Geometry check sheet. Reference: the model listing, model coordinates, mm. Round coordinates to 2 decimals unless told otherwise and drop trailing zeros. Loops run counter-clockwise (first coordinate to the right, second up) from the corner with the lowest first, then second, coordinate; pieces in that order, holes last. Notation, with made-up numbers: (-21.75, -12) - (-8.75, -12) arc R27 ccw to (-8.75, 13) - close; hole circle Ø3 at (42, -28). An arc over 180 degrees is marked (long way). Write item = value, one per line.
```python
from build123d import *

# Parameters (mm, degrees)
SKETCH1_R           = 2.75
BOSS_EXTRUDE1_DEPTH = 5.5


with BuildPart() as part:
    # Sketch1 → Boss-Extrude1 (new body)
    # profile 1 of 3: a face of its own
    with BuildSketch(Plane.XY):
        with BuildLine():
            ThreePointArc((-12.496095275, 0.312414586), (0, 12.5), (12.496095275, 0.312414586))
            Line((12.496095275, 0.312414586), (7.499414268, 400.093731696))
            ThreePointArc((7.499414268, 400.093731696), (0, 407.5), (-7.499414268, 400.093731696))
            Line((-7.499414268, 400.093731696), (-12.496095275, 0.312414586))
        make_face()
        with Locations((0, 400)):
            Circle(SKETCH1_R, mode=Mode.SUBTRACT)
    # profile 2 of 3: a face of its own
    with BuildSketch(Plane.XY):
        with BuildLine():
            ThreePointArc((-4.2, 0), (0, 4.2), (4.2, 0))
            Line((4.2, 0), (12.5, 0))
            Line((12.5, 0), (12.496095275, 0.312414586))
            ThreePointArc((12.496095275, 0.312414586), (0, 12.5), (-12.496095275, 0.312414586))
            Line((-12.496095275, 0.312414586), (-12.5, 0))
            Line((-12.5, 0), (-4.2, 0))
        make_face()
    # profile 3 of 3: a face of its own
    with BuildSketch(Plane.XY):
        with BuildLine():
            Line((12.5, 0), (4.2, 0))
            ThreePointArc((4.2, 0), (0, -4.2), (-4.2, 0))
            Line((-4.2, 0), (-12.5, 0))
            ThreePointArc((-12.5, 0), (0, -12.5), (12.5, 0))
        make_face()
    extrude(amount=BOSS_EXTRUDE1_DEPTH)


solid = part.part
```
(1) Section check B-B (y = 300.5). Enter the section's corners in (x, z).
Answers follow:
outline = (-8.74, 0) - (8.74, 0) - (8.74, 5.5) - (-8.74, 5.5) - close
(2) Section check C-C (y = 209). Enter the section's corners in (x, z).
Answers follow:
outline = (-9.89, 0) - (9.89, 0) - (9.89, 5.5) - (-9.89, 5.5) - close
(3) Scan lines: L1, parallel to Y at x = 0.5, z = 3.3; L2, parallel to X at y = 400, z = 2.65; L3, parallel to Y at x = -1, z = 0.55. Record each from-to range of solid material in increasing order. Write a range as [from, to].
Answers follow:
L1 = [-12.49, -4.17], [4.17, 397.3], [402.7, 407.48]
L2 = [-7.5, -2.75], [2.75, 7.5]
L3 = [-12.46, -4.08], [4.08, 397.44], [402.56, 407.43]
(4) Mould release check, pull along Y, two halves, no side actions. Record for faces 1 (the cylindrical face through (0.16, 407.5, 2.71)), 2 (the cylindrical face through (-0.547, -4.164, 2.712)), 3 (the flat face through (0, 200, 0)): pulls with the +Y half, pulls with the -Y half, needs draft (parallel to the pull), parting line crosses it, or undercut.
Answers follow:
face_1 = pulls with the +Y half
face_2 = undercut
face_3 = needs draft
(5) Section check A-A (z = 4.1). Enter the section's corners in (x, y), then the cut area to 3 significant figures.
Answers follow:
outline = (-12.5, 0) arc R12.5 ccw to (12.5, 0) - (7.5, 400.09) arc R7.5 ccw to (-7.5, 400.09) - close; hole circle Ø8.4 at (0, 0); hole circle Ø5.5 at (0, 400)
area = 8,250 mm²
